```python
from build123d import *

# Parameters (mm, degrees)
PAD001_DEPTH    = 15
SKETCH003_R     = 2
POCKET001_DEPTH = 5
FILLET001_R     = 1
CHAMFER001_SIZE = 1


with BuildPart() as part:
    # Sketch002 → Pad001 (new body)
    with BuildSketch(Plane.XY):
        with BuildLine():
            Line((-35, 15), (0, 15))
            Line((0, 15), (0, 0))
            Line((0, 0), (-5, 0))
            Line((-5, 0), (-5, 10))
            Line((-5, 10), (-35, 10))
            ThreePointArc((-35, 10), (-42.5, 2.5), (-35, -5))
            Line((-35, -5), (13, -5))
            Line((13, -5), (13, -34))
            Line((13, -34), (-22, -34))
            Line((-22, -34), (-22, -29))
            Line((-22, -29), (8, -29))
            Line((8, -29), (8, -10))
            Line((8, -10), (-35, -10))
            ThreePointArc((-35, 15), (-47.5, 2.5), (-35, -10))
        make_face()
    extrude(amount=PAD001_DEPTH)

    # Sketch003 (on Face9 of Pad001) → Pocket001 (cut)
    with BuildSketch(Plane.XZ.offset(34)):
        with Locations((-2, 7.5)):
            Circle(SKETCH003_R)
    extrude(amount=-POCKET001_DEPTH, mode=Mode.SUBTRACT)

    # Fillet001
    fillet001_edges = [part.edges().sort_by_distance(p)[0] for p in [
        (-22, -29, 7.5),
        (-22, -34, 7.5),
        (-4.5, -34, 15),
        (-7, -29, 15),
        (-7, -29, 0),
        (13, -19.5, 15),
        (8, -19.5, 15),
        (-13.5, -10, 15),
        (-47.5, 2.5, 15),
        (-42.5, 2.5, 15),
        (-47.5, 2.5, 0),
        (-17.5, 15, 0),
        (-17.5, 15, 15),
        (0, 15, 7.5),
        (0, 7.5, 15),
        (-20, 10, 15),
        (-42.5, 2.5, 0),
        (-11, -5, 0),
        (-5, 5, 15),
        (-5, 0, 7.5),
        (13, -5, 7.5),
        (-2.5, 0, 15),
        (8, -29, 7.5),
        (8, -10, 7.5),
        (8, -19.5, 0),
        (-22, -31.5, 15),
        (-22, -31.5, 0),
        (-20, 10, 0),
        (-5, 5, 0),
        (-2.5, 0, 0),
        (-13.5, -10, 0),
        (-4.5, -34, 0),
        (13, -19.5, 0),
    ]]
    fillet(fillet001_edges, radius=FILLET001_R)

    # Chamfer001
    chamfer001_edges = [part.edges().sort_by_distance(p)[0] for p in [
        (-4, -34, 7.5),
    ]]
    chamfer(chamfer001_edges, length=CHAMFER001_SIZE)


solid = part.part
```
Source: CAD feature listing. Evaluate the final solid. Frame: model axes, mm. A direction names the side the tool comes from. Coordinates: 2 decimals unless noted, no trailing zeros. Loops run counter-clockwise (first coordinate to the right, second up) from the corner with the lowest first, then second, coordinate; pieces in that order, holes last. Notation, with made-up numbers: (59.25, 48.25) -> (70.25, 48.25) arc R7 ccw to (70.25, 56.25) -> close; hole circle Ø7 at (69.25, -21). An arc over 180 degrees is marked (long way). One line per item, written item: value. Start each with the question number.
Q1. Set-up query: faces 1 (the face through (8, -20, 7)), 2 (the face through (-22, -32, 7)), 3 (the face through (-12, -5, 7)), 4 (the face through (-42.5, 2.66, 7.41)), 5 (the face through (-2.26, -31.028, 9.483)). Return all of +Z, -Z, +X, -X, +Y, -Y with unobstructed straight access to the full face (end or side cutting, diameter ignored); none if empty.
Q2. Contact query for flat-ended pins moving along their axis: P1, Ø8, axis at x = -27, y = -28.5, coming from the -Z side; P2, Ø4, axis at y = -8, z = 5, coming from the -X side; P3, Ø4, axis at y = -19, z = 8.5, coming from the -X side; P4, Ø7, axis at y = 6.5, z = 4, coming from the +X side. Output: stop coordinate, or through.
Q3. Section query B-B, the plane x = -2. Give the number of separate pieces and of enclosed holes in the cut face, and give its area (3 significant figures).
Q4. Mould query, pull axis X, two halves, no side actions, for faces 6 (the face through (0, 7, 7)), 7 (the face through (-5, 5, 7)), 8 (the face through (-47.497, 2.775, 7.409)). Classes: pulls with the +X half, pulls with the -X half, needs draft (parallel to the pull), parting line crosses it, or undercut.
Q5. Section query D-D, the plane y = -21. Return the cut outline in (x, z).
Q6. Section query A-A, the plane x = -24.5. Return the cut outline in (y, z), and give its area (3 significant figures).
Q7. Line query: line 1 along Y through (x, z) = (-14.5, 1.25); line 2 along Z through (x, y) = (-2, -32); line 3 along Y through (x, z) = (-25.5, 13.25). Output: solid intervals per line, ascending.
Q8. Section query C-C, the plane z = 7.5. Return the cut outline in (x, y).
Results:
1. face 1: +Z, -Z, -X
1. face 2: +Z, -Z, -X, -Y
1. face 3: +Z, -Z, +X
1. face 4: +Z, -Z
1. face 5: -Y
2. P1: through
2. P2: x = -44.17
2. P3: x = 8
2. P4: x = 0
3. separate pieces: 4
3. enclosed holes: 0
3. area: 351 mm^2
4. face 6: pulls with the +X half
4. face 7: undercut
4. face 8: pulls with the -X half
5. outline: (8, 1) arc R1 ccw to (9, 0) -> (12, 0) arc R1 ccw to (13, 1) -> (13, 14) arc R1 ccw to (12, 15) -> (9, 15) arc R1 ccw to (8, 14) -> close
6. outline: (-10, 1) arc R1 ccw to (-9, 0) -> (-6, 0) arc R1 ccw to (-5, 1) -> (-5, 14) arc R1 ccw to (-6, 15) -> (-9, 15) arc R1 ccw to (-10, 14) -> close; (10, 1) arc R1 ccw to (11, 0) -> (14, 0) arc R1 ccw to (15, 1) -> (15, 14) arc R1 ccw to (14, 15) -> (11, 15) arc R1 ccw to (10, 14) -> close
6. area: 148 mm^2
7. line 1: -34 to -29, -10 to -5, 10 to 15
7. line 2: 0 to 5.5, 9.5 to 15
7. line 3: -10 to -5, 10 to 15
8. outline: (-35, -10) -> (7, -10) arc R1 cw to (8, -11) -> (8, -28) arc R1 cw to (7, -29) -> (0, -29) -> (0, -33) -> (1, -34) -> (13, -34) -> (13, -6) arc R1 ccw to (12, -5) -> (-35, -5) arc R7.5 cw to (-35, 10) -> (-5, 10) -> (-5, 1) arc R1 ccw to (-4, 0) -> (0, 0) -> (0, 14) arc R1 ccw to (-1, 15) -> (-35, 15) arc R12.5 ccw to start; (-22, -33) arc R1 ccw to (-21, -34) -> (-5, -34) -> (-4, -33) -> (-4, -29) -> (-21, -29) arc R1 ccw to (-22, -30) -> close
